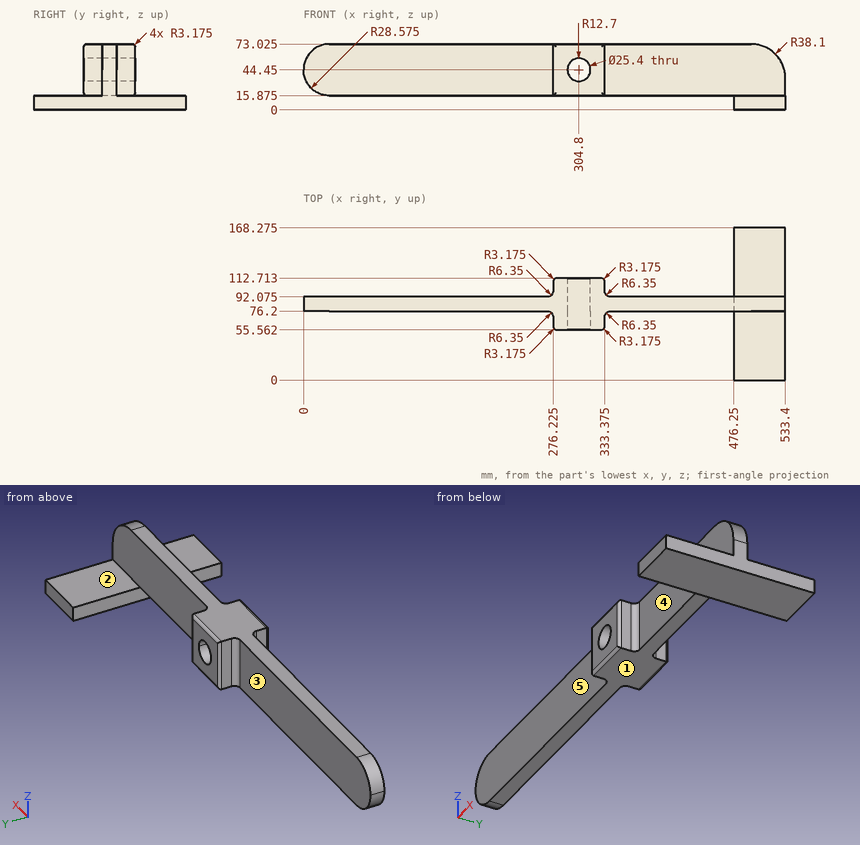
Job drawing, mm, ordinate dimensions from the low corner. One solid piece. A direction names the side the tool comes from. Give positions to 0.01 mm unless a question says otherwise; leave off trailing zeros. Use one line per item in the form item = value. Start each with the question number.
1. Drop flat-ended pins along their axis: pin 1 Ø17 at (x, z) = (132, 42.5) entering from +Y (1 decimal); pin 2 Ø5 at (y, z) = (108, 9) entering from -X; pin 3 Ø9 at (y, z) = (102.5, 39.5) entering from +X. Give the stop position or say it passes through.
2. 3-axis set-ups, long thin cutter, end or side, ignore diameter. For the marked faces 1, 2, 3, 4 and 5: which of +Z, -Z, +X, -X, +Y, -Y reach the whole face in a straight line?
3. Probe line 1 (X direction, y = 60.25, z = 44.45) (1 decimal); line 2 (Y direction, x = 218, z = 67) (1 decimal); line 3 (X direction, y = 86.5, z = 9). List the from-to ranges inside material, lowest first. Write a range as [from, to].
Conclusion:
q1.pin_1 = 92.1
q1.pin_2 = 476.25
q1.pin_3 = 333.39
q2.face_1 = -Z, -X, +Y, -Y
q2.face_2 = +Z, +X, +Y
q2.face_3 = +Z, -Z, -X, +Y
q2.face_4 = +Z, +X, -Y
q2.face_5 = +Z, -Z, -X, -Y
q3.line_1 = [276.2, 292.1], [317.5, 333.4]
q3.line_2 = [76.2, 92.1]
q3.line_3 = [476.25, 533.4]
